Autodesk Inventor part; units mm, degrees
ref_plane "YZ Plane" through (0, 0, 0) normal (1, 0, 0) x (0, 1, 0)
ref_plane "XZ Plane" through (0, 0, 0) normal (0, 1, 0) x (-1, 0, 0)
ref_plane "XY Plane" through (0, 0, 0) normal (0, 0, 1) x (1, 0, 0)
sketch "Sketch1" plane through (0, 0, 0) normal (0, 1, 0) x (-1, 0, 0)
  line L0 (0, 279.3478) -> (-39.1304, 279.3478)
  line L1 (-39.1304, 279.3478) -> (-39.1304, -270.6522)
  line L2 (-39.1304, -270.6522) -> (0, -270.6522)
  line L3 (0, -270.6522) -> (0, 279.3478)
  line L4 (-39.1304, 279.3478) -> (-29.1304, 279.3478)
  line L5 (-29.1304, 254.3478) -> (-39.1304, 254.3478)
  line L6 (-39.1304, 254.3478) -> (-39.1304, 279.3478)
  line L7 (-39.1304, -270.6522) -> (-29.1304, -270.6522)
  line L8 (-29.1304, -245.6522) -> (-39.1304, -245.6522)
  line L9 (-39.1304, -245.6522) -> (-39.1304, -270.6522)
  point P0 (0, 0)
  point P1 (-39.1304, 254.3478)
  point P2 (-39.1304, -245.6522)
  dimension "d0" = 550
  dimension "d4" = 25
  dimension "d5" = 25
  dimension "d28" = 39.1304
extrude "Extrusion1" add sketch "Sketch1" along normal blind 160
sketch "Sketch2" plane through (0, 0, 279.3478) normal (0, 0, 1) x (1, 0, 0)
  line L0 (0, 160) -> (39.1304, 160)
  line L1 (0, 160) -> (39.1304, 160)
  line L2 (39.1304, 160) -> (39.1304, 0)
  line L3 (39.1304, 0) -> (0, 0)
  line L4 (0, 0) -> (0, 160)
  line L5 (39.1304, 160) -> (29.1304, 160)
  line L6 (29.1304, 160) -> (29.1304, 115)
  line L7 (29.1304, 115) -> (39.1304, 115)
  line L8 (39.1304, 115) -> (39.1304, 160)
  line L9 (39.1304, 0) -> (29.1304, 0)
  line L10 (29.1304, 0) -> (29.1304, 45)
  line L11 (29.1304, 45) -> (39.1304, 45)
  line L12 (39.1304, 45) -> (39.1304, 0)
  circle A0 centre (39.1304, 80) radius 18
  line L13 (21.1304, 75) -> (39.1304, 75)
  line L14 (39.1304, 75) -> (39.1304, 98)
  line L15 (39.1304, 98) -> (21.1304, 98)
  line L16 (21.1304, 98) -> (21.1304, 75)
  line L17 (21.1304, 75) -> (39.1304, 75)
  line L18 (39.1304, 75) -> (39.1304, 62)
  line L19 (39.1304, 62) -> (21.1304, 62)
  line L20 (21.1304, 62) -> (21.1304, 75)
  line L21 (39.1304, 0) -> (39.1304, 160)
  line L22 (0, 160) -> (9.1304, 160)
  line L23 (9.1304, 160) -> (9.1304, 0)
  line L24 (9.1304, 0) -> (0, 0)
  line L25 (0, 0) -> (0, 160)
  point P0 (0, 0)
  point P1 (34.1304, 115)
  point P2 (34.1304, 160)
  point P3 (39.1304, 45)
  point P4 (39.1304, 115)
  dimension "d6" = 10
  dimension "d7" = 45
  dimension "d8" = 45
  dimension "d9" = 18
  dimension "d10" = 36
  dimension "d11" = 80
  dimension "d12" = 80
  dimension "d15" = 30
extrude "Extrusion2" cut sketch "Sketch2" against normal up to surface (550 mm away) contours L0 L23 L3 L4 | L0 L2 L7 L6 | L10 L11 L2 L3 | L2 L13 A0 | A0 L16 L15 | L2 A0 L13 | A0 L13 L16 | L19 L20 L13 A0
sketch "Sketch3" plane through (21.1304, 62, 279.3478) normal (1, 0, 0) x (0, 0, -1)
  line L0 (550, 0) -> (0, 0)
  line L1 (0, 0) -> (0, 36)
  line L2 (0, 36) -> (550, 36)
  circle A0 centre (54, 18) radius 10
  circle A1 centre (104, 18) radius 10
  circle A2 centre (154, 18) radius 10
  circle A3 centre (204, 18) radius 10
  circle A4 centre (254, 18) radius 10
  circle A5 centre (304, 18) radius 10
  circle A6 centre (354, 18) radius 10
  circle A7 centre (404, 18) radius 10
  circle A8 centre (454, 18) radius 10
  point P0 (279.3478, -62)
  dimension "d18" = 50
extrude "Extrusion3" cut sketch "Sketch3" against normal blind 25 contours A0 | A1 | A2 | A3 | A4 | A5 | A6 | A7
chamfer "Chamfer1" distance 8 distance2 5 8 edges at (21.1304, 80, 235.3478) (21.1304, 80, 185.3478) (21.1304, 80, 135.3478) (21.1304, 80, 85.3478) (21.1304, 80, 35.3478) (21.1304, 80, -14.6522) (21.1304, 80, -64.6522) (21.1304, 80, -114.6522) measured on face at (21.1304, 80, -225.3188)
properties part number "MainRails" material "Aluminum 6061"
Check sheet for the modelled part. Datum: model origin and axes. Units: mm. A direction names the side the tool comes from. Round coordinates to 2 decimals unless told otherwise and drop trailing zeros. Order: outer loops, then holes, each group sorted by start corner. A loop starts at its lowest first (then second) coordinate and runs counter-clockwise, first axis right, second up.
1) Tool access check on faces 1 (the flat face through (29.13, 22, 8)), 2 (the cylindrical face through (12.68, 88.43, -30.03)). Record the directions out of +Z, -Z, +X, -X, +Y, -Y that give a thin tool (end or side, any length) a straight path to the whole face; none if there is none.
2) Section check B-B (y = 80). Give the number of separate pieces and of enclosed holes in the cut face, and give its area (3 significant figures).
3) Scan lines: line 1 (Y direction, x = 21.25, z = -144.5); line 2 (Y direction, x = 36.5, z = -135.5); line 3 (X direction, y = 120.5, z = 87). Record each from-to range of solid material in increasing order.
4) Go/stop test with flat-tipped pins: pin 1 Ø8 at (x, z) = (35, -60) entering from +Y; pin 2 Ø3 at (x, z) = (31.5, 30) entering from -Y; pin 3 Ø16 at (y, z) = (80, 175.35) entering from +X; pin 4 Ø11 at (y, z) = (75, -33) entering from +X. Record where each tip stops, or that it passes through.
5) Mould release check, pull along Y, two halves, no side actions. Record for faces 3 (the cylindrical face through (12.68, 83, -134.19)), 4 (the flat face through (21.13, 80, -53)), 5 (the flat face through (19, 160, 8)), 6 (the flat face through (20.6, 78.9, 279.348)): +Y half, -Y half, draft (parallel to the pull), parting line (faces both ways), or undercut.
6) Section check C-C (y = 122). Record the boundary of the cut face in (x, z).
7) Section check A-A (z = -196.5). Record the boundary of the cut face in (x, y).
Result:
1. face 1: +Z, -Z, +X, -Y
1. face 2: +X, -X
2. separate pieces: 9
2. enclosed holes: 0
2. area: 4,360 mm2
3. line 1: y = 0 to 62, 98 to 160
3. line 2: y = 45 to 62, 98 to 115
3. line 3: x = 9.13 to 29.13
4. pin 1: stops at y = 115
4. pin 2: stops at y = 45
4. pin 3: passes through
4. pin 4: stops at x = 19.4
5. face 3: undercut
5. face 4: undercut
5. face 5: +Y half
5. face 6: draft
6. outline: (9.13, -270.65) - (29.13, -270.65) - (29.13, 279.35) - (9.13, 279.35) - close
7. outline: (9.13, 0) - (29.13, 0) - (29.13, 45) - (39.13, 45) - (39.13, 62) - (21.13, 62) - (21.13, 98) - (39.13, 98) - (39.13, 115) - (29.13, 115) - (29.13, 160) - (9.13, 160) - close
